from build123d import *

# Parameters (mm, degrees)
SKETCH1_W           = 20
SKETCH1_H           = 20
SKETCH1_R           = 1.5
BOSS_EXTRUDE1_DEPTH = 5
SKETCH2_R           = 1.75
BOSS_EXTRUDE2_DEPTH = 5
SKETCH3_R           = 1.75
BOSS_EXTRUDE3_DEPTH = 5
FILLET1_R           = 17


with BuildPart() as part:
    # Sketch1 → Boss-Extrude1 (new body)
    with BuildSketch(Plane(origin=(0, 0, 0), x_dir=(1, 0, 0), z_dir=(0, 1, 0))):
        with Locations((10, 10)):
            Rectangle(SKETCH1_W, SKETCH1_H)
        with Locations(Location((10, 15, 0), (0, 0, 270))):
            Circle(SKETCH1_R, mode=Mode.SUBTRACT)
        with Locations(Location((15, 10, 0), (0, 0, 270))):
            Circle(SKETCH1_R, mode=Mode.SUBTRACT)
    extrude(amount=BOSS_EXTRUDE1_DEPTH)

    # Sketch2 → Boss-Extrude2 (add)
    with BuildSketch(Plane.XY):
        with BuildLine():
            Line((19, 0), (5, 0))
            ThreePointArc((5, 0), (12, -7), (19, 0))
        make_face()
        with Locations((12, -4)):
            Circle(SKETCH2_R, mode=Mode.SUBTRACT)
    extrude(amount=-BOSS_EXTRUDE2_DEPTH)

    # Sketch3 → Boss-Extrude3 (add)
    with BuildSketch(Plane.ZY):
        with BuildLine():
            Line((0, 0), (-14, 0))
            ThreePointArc((-14, 0), (-7, -7), (0, 0))
        make_face()
        with Locations((-7, -4)):
            Circle(SKETCH3_R, mode=Mode.SUBTRACT)
    extrude(amount=-BOSS_EXTRUDE3_DEPTH)

    # Fillet1
    fillet1_edges = [part.edges().sort_by_distance(p)[0] for p in [
        (20, 2.5, -20),
    ]]
    fillet(fillet1_edges, radius=FILLET1_R)


solid = part.part
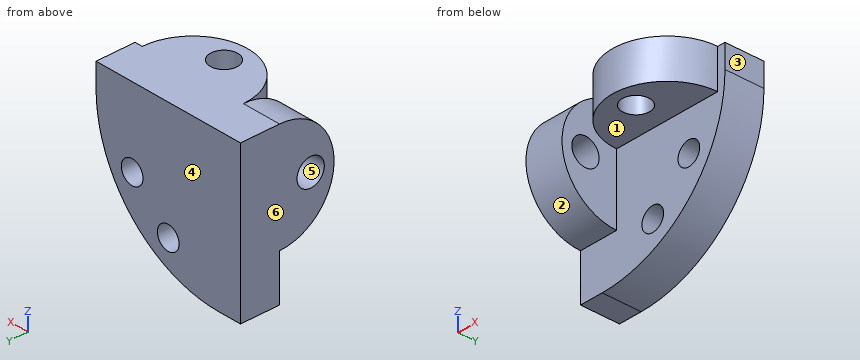
The model under review builds one solid part; all positions refer to its coordinate system, in mm. Face numbers are marked on the shaded views. A direction names the side the tool comes from. Coordinates: 2 decimals unless noted, no trailing zeros. Loops run counter-clockwise (first coordinate to the right, second up) from the corner with the lowest first, then second, coordinate; pieces in that order, holes last. Notation, with made-up numbers: M 70.5,73 L 101.5,73 A27 ccw 101.5,90 Z; hole C 28,67 d10. An arc over 180 degrees is marked long. Put each result on its own line as item: value. Start each with the question number.
Q1. Wall thickness on line 1 (Y direction, x = 8.5, z = -8.25); line 2 (Y direction, x = 12, z = -2.75); line 3 (X direction, y = 3.7, z = -15): over which ranges is each line inside the solid? List them lowest first.
Q2. Add section C-C (x = 1.5). Write out the cut boundary in (y, z), and give its area (3 significant figures).
Q3. The part is to be moulded in two halves that separate along Y. For the marked faces 4, 5 and 6, say which applies: +Y half, -Y half, draft (parallel to the pull), parting line (faces both ways), or undercut.
Q4. Add section A-A (y = -4.75). Write out the cut boundary in (x, z), and give its area (3 significant figures).
Q5. For the marked faces 1, 2 and 3, list the 3-axis set-ups (+Z, -Z, +X, -X, +Y, -Y) from which the entire face can be reached by the end or side of a thin tool; tool diameter is ignored.
Q6. Add section D-D (x = 9). Write out the cut boundary in (y, z), and give its area (3 significant figures).
Q7. Add section B-B (z = -9.25). Write out the cut boundary in (x, y), and give its area (3 significant figures).
Q8. Clearance check with flat-ended pins moving along their axes: pin 1 (8 mm diameter, centred on x = 5.5, z = -8, fed in from -Y); pin 2 (2 mm diameter, centred on x = 12, y = -4, fed in from +Z); pin 3 (3.5 mm diameter, centred on x = 10.5, y = -3.5, fed in from -Z); pin 4 (1 mm diameter, centred on x = 11, z = -14.5, fed in from -Y). State where each tip first meets the part, or that it passes through.
Answers:
1. line 1: y = 0 to 5
1. line 2: y = -7 to -5.75, -2.25 to 5
1. line 3: x = 0 to 8.5, 11.5 to 15.04
2. outline: M 0,-20 L 5,-20 L 5,0 L 0,0 A7 ccw 0,-14 Z; hole C -4,-7 d3.5
2. area: 167 mm^2
3. face 4: +Y half
3. face 5: undercut
3. face 6: draft
4. outline: M 0,-12.14 L 5,-12.14 L 5,-8.58 L 0,-8.58 Z; M 0,-5.42 L 5,-5.42 L 5,-1.86 L 0,-1.86 Z; M 6.86,-5 L 10.42,-5 L 10.42,0 L 6.86,0 Z; M 13.58,-5 L 17.14,-5 L 17.14,0 L 13.58,0 Z
4. area: 71.2 mm^2
5. face 1: -Z, +X, -Y
5. face 2: -X, -Y
5. face 3: +Z, -Z, +X, +Y, -Y
6. outline: M -6.32,-5 L 0,-5 L 0,-13.88 L 5,-13.88 L 5,0 L -6.32,0 Z; M 0,-18.91 L 5,-18.91 L 5,-16.12 L 0,-16.12 Z
6. area: 115 mm^2
7. outline: M 0,-6.63 L 5,-6.63 L 5,0 L 13.7,0 L 13.7,5 L 0,5 Z; M 16.3,0 L 18.81,0 L 18.81,5 L 16.3,5 Z
7. area: 114 mm^2
8. pin 1: stops at y = -7
8. pin 2: passes through
8. pin 3: stops at z = -5
8. pin 4: stops at y = 0
